Part print with two shaded views. Sizes in mm from the minimum x, y, z corner. A direction names the side the tool comes from. Give positions to 0.01 mm unless a question says otherwise; leave off trailing zeros. Write each loop counter-clockwise with the first axis right and the second up, starting at its lowest first coordinate (ties: lowest second). Pieces come first, ordered by that corner, then holes. Notation, with made-up numbers: (7, 13.5) - (42, 13.5) arc R4 cw to (42, 20.5) - close; hole circle Ø11 at (-24, -29.75). An arc over 180 degrees is marked (long way). One line per item, written item: value. Start each with the question number.
(1) Mould opens along X. For the marked faces 4, 5 and 6 say: pulls with the +X half, pulls with the -X half, needs draft (parallel to the pull), parting line crosses it, or undercut.
(2) Cut at D-D, the plane x = 2.75. List the corners of the cut face in (y, z).
(3) 3-axis set-ups, long thin cutter, end or side, ignore diameter. For the marked faces 1, 2 and 3: which of +Z, -Z, +X, -X, +Y, -Y reach the whole face in a straight line?
(4) Cut at A-A, the plane x = 7. List the corners of the cut face in (y, z).
(5) Cut at C-C, the plane y = 10.25. List the corners of the cut face in (x, z), and give its area (3 significant figures).
(6) Probe L1, parallel to X at y = 4, z = 17.5; L2, parallel to Z at x = 3.5, y = 9.75; L3, parallel to Z at x = 3.75, y = 1.75. List the from-to ranges inside material, lowest first.
(7) Cut at B-B, the plane z = 12.75. List the corners of the cut face in (x, y).
(8) Drop flat-ended pins along their axis: P1, Ø8, axis at x = 8, z = 13.5, coming from the -Y side; P2, Ø1.4, axis at y = 7.5, z = 5, coming from the +X side; P3, Ø4, axis at y = 7, z = 9, coming from the -X side; P4, Ø4, axis at y = 11, z = 11.5, coming from the +X side. Give the stop position or say it passes through.
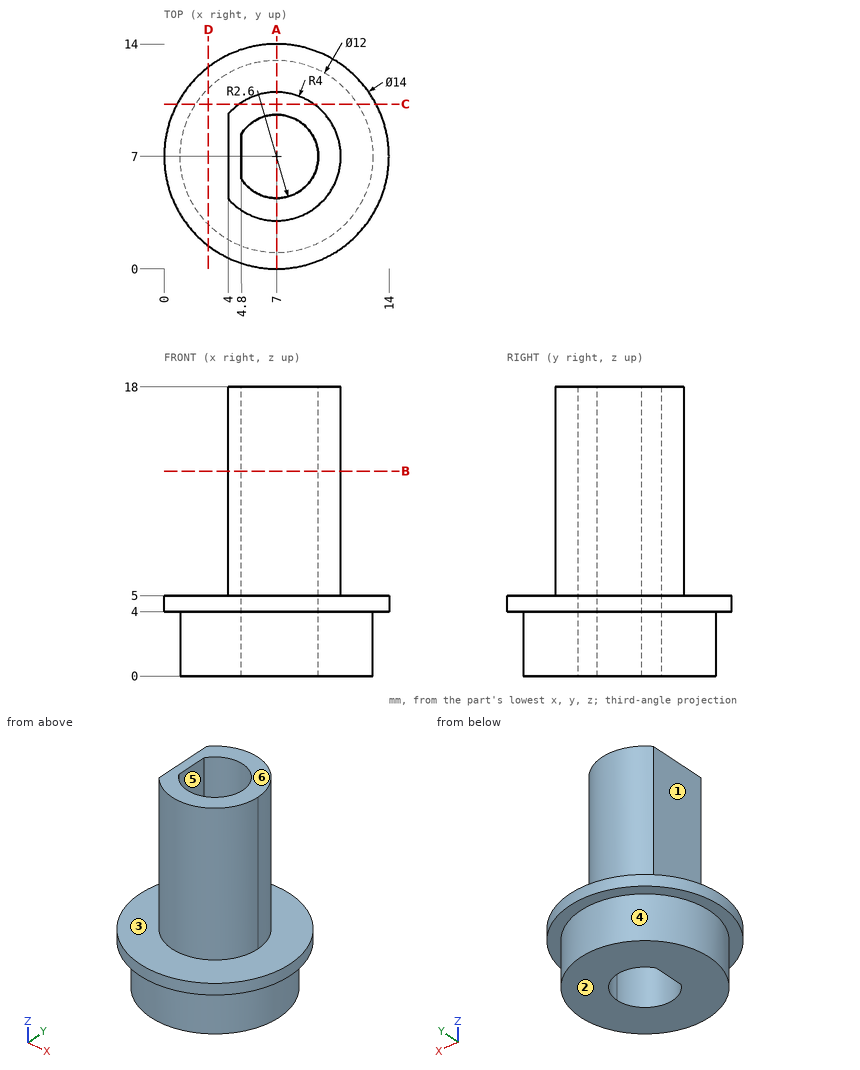
Answers follow:
1. face 4: parting line crosses it
1. face 5: undercut
1. face 6: needs draft
2. outline: (1.44, 4) - (2.76, 4) - (2.76, 0) - (11.24, 0) - (11.24, 4) - (12.56, 4) - (12.56, 5) - (1.44, 5) - close
3. face 1: +Z, -X, +Y, -Y
3. face 2: -Z, +X, -X, +Y, -Y
3. face 3: +Z
4. outline: (0, 4) - (1, 4) - (1, 0) - (4.4, 0) - (4.4, 18) - (3, 18) - (3, 5) - (0, 5) - close; (9.6, 0) - (13, 0) - (13, 4) - (14, 4) - (14, 5) - (11, 5) - (11, 18) - (9.6, 18) - close
5. outline: (0.8, 4) - (1.96, 4) - (1.96, 0) - (12.04, 0) - (12.04, 4) - (13.2, 4) - (13.2, 5) - (9.33, 5) - (9.33, 18) - (4.67, 18) - (4.67, 5) - (0.8, 5) - close
5. area: 113 mm²
6. L1: x = 4.35 to 9.65
6. L2: z = 0 to 5
6. L3: z = 4 to 5
7. outline: (4, 4.35) arc R4 ccw (long way) to (4, 9.65) - close; hole (4.8, 5.61) arc R2.6 ccw (long way) to (4.8, 8.39) - close
8. P1: stops at y = 3
8. P2: stops at x = 14
8. P3: stops at x = 4
8. P4: stops at x = 10.46
